For this review, take the finished solid that the model builds, in its own axes (mm). A direction names the side the tool comes from. Round coordinates to 2 decimals unless told otherwise and drop trailing zeros. Order: outer loops, then holes, each group sorted by start corner. A loop starts at its lowest first (then second) coordinate and runs counter-clockwise, first axis right, second up. Notation, with made-up numbers: M 29,13.5 L 55,13.5 A8 ccw 55,18.5 Z; hole C -9.75,-23 d7. An arc over 180 degrees is marked long. Answer in a Markdown table with one row per item. Add a question column.
```python
from build123d import *

# Parameters (mm, degrees)
SKETCH1_R           = 73.65
SKETCH1_R_2         = 5.55625
BOSS_EXTRUDE1_DEPTH = 3
BOSS_EXTRUDE2_START = -3
SKETCH1_3_R         = 76.2
SKETCH1_3_R_2       = 73.65
SKETCH1_3_R_3       = 5.55625
BOSS_EXTRUDE2_DEPTH = 3


with BuildPart() as part:
    # Sketch1 → Boss-Extrude1 (new body)
    with BuildSketch(Plane(origin=(0, 0, 0), x_dir=(1, 0, 0), z_dir=(0, 1, 0))):
        with Locations(Location((0, 0, 0), (0, 0, 270))):
            Circle(SKETCH1_R)
        with Locations(Location((25.4, 0, 0), (0, 0, 270))):
            Circle(SKETCH1_R_2, mode=Mode.SUBTRACT)
        with Locations(Location((-25.4, 0, 0), (0, 0, 270))):
            Circle(SKETCH1_R_2, mode=Mode.SUBTRACT)
        with Locations(Location((0, 50, 0), (0, 0, 270))):
            Circle(SKETCH1_R_2, mode=Mode.SUBTRACT)
        with Locations(Location((0, -50, 0), (0, 0, 270))):
            Circle(SKETCH1_R_2, mode=Mode.SUBTRACT)
    extrude(amount=BOSS_EXTRUDE1_DEPTH)

    # Sketch1_3 → Boss-Extrude2 (add)
    # profile 1 of 2: a face of its own
    with BuildSketch(Plane(origin=(0, 0, 0), x_dir=(1, 0, 0), z_dir=(0, 1, 0)).offset(BOSS_EXTRUDE2_START)):
        with Locations(Location((0, 0, 0), (0, 0, 270))):
            Circle(SKETCH1_3_R)
        with Locations(Location((0, 0, 0), (0, 0, 270))):
            Circle(SKETCH1_3_R_2, mode=Mode.SUBTRACT)
    # profile 2 of 2: a face of its own
    with BuildSketch(Plane(origin=(0, 0, 0), x_dir=(1, 0, 0), z_dir=(0, 1, 0)).offset(BOSS_EXTRUDE2_START)):
        with Locations(Location((0, 0, 0), (0, 0, 270))):
            Circle(SKETCH1_3_R_2)
        with Locations(Location((25.4, 0, 0), (0, 0, 270))):
            Circle(SKETCH1_3_R_3, mode=Mode.SUBTRACT)
        with Locations(Location((-25.4, 0, 0), (0, 0, 270))):
            Circle(SKETCH1_3_R_3, mode=Mode.SUBTRACT)
        with Locations(Location((0, 50, 0), (0, 0, 270))):
            Circle(SKETCH1_3_R_3, mode=Mode.SUBTRACT)
        with Locations(Location((0, -50, 0), (0, 0, 270))):
            Circle(SKETCH1_3_R_3, mode=Mode.SUBTRACT)
    extrude(amount=BOSS_EXTRUDE2_DEPTH)


solid = part.part
```
1. The part is to be moulded in two halves that separate along Z. For faces 1 (the flat face through (1, 3, -1)), 2 (the cylindrical face through (0.24, -0.04, -55.55)), 3 (the cylindrical face through (22.12, 1.48, 70.25)), 4 (the cylindrical face through (30.91, -0.04, -0.72)), say which applies: pulls with the +Z half, pulls with the -Z half, needs draft (parallel to the pull), parting line crosses it, or undercut.
2. Consider section D-D on z = -50. Write out the cut boundary in (x, y), plus the area to 3 significant figures.
3. To check wall thickness, follow probe 1 along X at (y, z) = (-1.4, 0); probe 2 along X at (y, z) = (0.25, 50); probe 3 along Y at (x, z) = (51, -54). State the ranges of each line that lie inside material, in increasing order. Write a range as [from, to].
4. Clearance check with flat-ended pins moving along their axes: pin 1 Ø1 at (x, y) = (-7, -1.5) entering from +Z; pin 2 Ø18 at (x, z) = (25.4, 0) entering from +Y; pin 3 Ø3 at (y, z) = (1, 22) entering from +X; pin 4 Ø2 at (y, z) = (0.5, 7.5) entering from +X. State where each tip first meets the part, or that it passes through.
5. Consider section A-A on x = 0. Write out the cut boundary in (y, z), plus the area to 3 significant figures.
6. Consider section C-C on y = -1.25. Write out the cut boundary in (x, z), plus the area to 3 significant figures.
7. For faces 5 (the cylindrical face through (-30.824, -0.042, -1.204)), 6 (the flat face through (62.4, 0, -39.9)), list the 3-axis set-ups (+Z, -Z, +X, -X, +Y, -Y) from which the entire face can be reached by the end or side of a thin tool; tool diameter is ignored.
8. Consider section B-B on x = 25.4. Write out the cut boundary in (y, z).
Solved:
| question | item | result |
|---|---|---|
| 1 | face 1 | needs draft |
| 1 | face 2 | undercut |
| 1 | face 3 | parting line crosses it |
| 1 | face 4 | undercut |
| 2 | outline | M -57.5,-3 L -5.56,-3 L -5.56,3 L -54.08,3 L -54.08,0 L -57.5,0 Z; M 5.56,-3 L 57.5,-3 L 57.5,0 L 54.08,0 L 54.08,3 L 5.56,3 Z |
| 2 | area | 603 mm^2 |
| 3 | probe 1 | x = [-76.2, -30.96], [-19.84, 19.84], [30.96, 76.2] |
| 3 | probe 2 | x = [-54.08, -5.56], [5.56, 54.08] |
| 3 | probe 3 | y = [-3, 0] |
| 4 | pin 1 | stops at z = 75.92 |
| 4 | pin 2 | stops at y = 3 |
| 4 | pin 3 | stops at x = 73.28 |
| 4 | pin 4 | stops at x = 75.91 |
| 5 | outline | M -3,-76.2 L 0,-76.2 L 0,-73.65 L 3,-73.65 L 3,-55.56 L -3,-55.56 Z; M -3,-44.44 L 3,-44.44 L 3,44.44 L -3,44.44 Z; M -3,55.56 L 3,55.56 L 3,73.65 L 0,73.65 L 0,76.2 L -3,76.2 Z |
| 5 | area | 766 mm^2 |
| 6 | outline | C 0,0 d152.4; hole C -25.4,0 d11.11; hole C 0,-50 d11.11; hole C 0,50 d11.11; hole C 25.4,0 d11.11 |
| 6 | area | 17,900 mm^2 |
| 7 | face 5 | +Y, -Y |
| 7 | face 6 | +Y |
| 8 | outline | M -3,-71.84 L 0,-71.84 L 0,-69.13 L 3,-69.13 L 3,-5.56 L -3,-5.56 Z; M -3,5.56 L 3,5.56 L 3,69.13 L 0,69.13 L 0,71.84 L -3,71.84 Z |
